```python
from build123d import *

# Parameters (mm, degrees)
SKETCH1_W           = 80
SKETCH1_H           = 40
BOSS_EXTRUDE1_DEPTH = 1.5
SKETCH3_W           = 6.333333333
SKETCH3_H           = 3
SKETCH3_W_2         = 12.666666667
CUT_EXTRUDE1_DEPTH  = 3
CUT_EXTRUDE3_DEPTH  = 3
SKETCH5_W           = 3
SKETCH5_H           = 8
CUT_EXTRUDE4_DEPTH  = 3
CUT_EXTRUDE6_DEPTH  = 3
FILLET1_R           = 3
BOSS_EXTRUDE2_START = -3
BOSS_EXTRUDE2_DEPTH = 3
FILLET2_R           = 6
BOSS_EXTRUDE3_START = -3
BOSS_EXTRUDE3_DEPTH = 3
FILLET3_R           = 1.5


with BuildPart() as part:
    # Sketch1 → Boss-Extrude1 (new body, symmetric)
    with BuildSketch(Plane.XY):
        with Locations((0, 5.625841184)):
            Rectangle(SKETCH1_W, SKETCH1_H)
    extrude(amount=BOSS_EXTRUDE1_DEPTH, both=True)

    # Sketch3 → Cut-Extrude1 (cut)
    with BuildSketch(Plane(origin=(0, 0, -1.5), x_dir=(-1, 0, 0), z_dir=(0, 0, -1))):
        with Locations((-36.833333334, 24.125841184)):
            Rectangle(SKETCH3_W, SKETCH3_H)
        with Locations((-13.333333334, 24.125841184)):
            Rectangle(SKETCH3_W_2, SKETCH3_H)
        with Locations((13.333333334, 24.125841184)):
            Rectangle(SKETCH3_W_2, SKETCH3_H)
        with Locations((36.833333334, 24.125841184)):
            Rectangle(SKETCH3_W, SKETCH3_H)
        with Locations((-36.833333334, -12.874158816)):
            Rectangle(SKETCH3_W, SKETCH3_H)
        with Locations((-13.333333334, -12.874158816)):
            Rectangle(SKETCH3_W_2, SKETCH3_H)
        with Locations((36.833333334, -12.874158816)):
            Rectangle(SKETCH3_W, SKETCH3_H)
        with Locations((13.333333334, -12.874158816)):
            Rectangle(SKETCH3_W_2, SKETCH3_H)
    extrude(amount=-CUT_EXTRUDE1_DEPTH, mode=Mode.SUBTRACT)

    # Sketch4 → Cut-Extrude3 (cut)
    with BuildSketch(Plane(origin=(0, 0, -1.5), x_dir=(-1, 0, 0), z_dir=(0, 0, -1))):
        Polygon((10.933333333, 17.875841184), (12.183333333, 17.875841184), (12.183333333, 15.625841184), (14.483333333, 15.625841184), (14.483333333, 17.875841184), (15.733333333, 17.875841184), (15.733333333, 19.625841184), (14.483333333, 19.625841184), (14.483333333, 22.625841184), (12.183333333, 22.625841184), (12.183333333, 19.625841184), (10.933333333, 19.625841184), align=None)
        Polygon((-12.183333333, 22.625841184), (-14.483333333, 22.625841184), (-14.483333333, 19.625841184), (-15.733333333, 19.625841184), (-15.733333333, 17.875841184), (-14.483333333, 17.875841184), (-14.483333333, 15.625841184), (-12.183333333, 15.625841184), (-12.183333333, 17.875841184), (-10.933333333, 17.875841184), (-10.933333333, 19.625841184), (-12.183333333, 19.625841184), align=None)
        Polygon((-10.933333333, -6.624158816), (-12.183333333, -6.624158816), (-12.183333333, -4.374158816), (-14.483333333, -4.374158816), (-14.483333333, -6.624158816), (-15.733333333, -6.624158816), (-15.733333333, -8.374158816), (-14.483333333, -8.374158816), (-14.483333333, -11.374158816), (-12.183333333, -11.374158816), (-12.183333333, -8.374158816), (-10.933333333, -8.374158816), align=None)
        Polygon((12.183333333, -11.374158816), (14.483333333, -11.374158816), (14.483333333, -8.374158816), (15.733333333, -8.374158816), (15.733333333, -6.624158816), (14.483333333, -6.624158816), (14.483333333, -4.374158816), (12.183333333, -4.374158816), (12.183333333, -6.624158816), (10.933333333, -6.624158816), (10.933333333, -8.374158816), (12.183333333, -8.374158816), align=None)
    extrude(amount=-CUT_EXTRUDE3_DEPTH, mode=Mode.SUBTRACT)

    # Sketch5 → Cut-Extrude4 (cut)
    with BuildSketch(Plane(origin=(0, 0, -1.5), x_dir=(-1, 0, 0), z_dir=(0, 0, -1))):
        with Locations((36.5, -4.374158816)):
            Rectangle(SKETCH5_W, SKETCH5_H)
        with Locations((36.5, 15.625841184)):
            Rectangle(SKETCH5_W, SKETCH5_H)
        with Locations((-36.5, 15.625841184)):
            Rectangle(SKETCH5_W, SKETCH5_H)
        with Locations((-36.5, -4.374158816)):
            Rectangle(SKETCH5_W, SKETCH5_H)
    extrude(amount=-CUT_EXTRUDE4_DEPTH, mode=Mode.SUBTRACT)

    # Sketch7 → Cut-Extrude6 (cut)
    with BuildSketch(Plane.XY.offset(1.5)):
        Polygon((-32, 19.625841184), (-32, -8.374158816), (-18.733333333, -8.374158816), (-18.733333333, -1.374158816), (-7.933333333, -1.374158816), (-7.933333333, -8.374158816), (7.933333333, -8.374158816), (7.933333333, -1.374158816), (18.733333333, -1.374158816), (18.733333333, -8.374158816), (32, -8.374158816), (32, 19.625841184), (18.733333333, 19.625841184), (18.733333333, 12.625841184), (7.933333333, 12.625841184), (7.933333333, 19.625841184), (-7.933333333, 19.625841184), (-7.933333333, 12.625841184), (-18.733333333, 12.625841184), (-18.733333333, 19.625841184), align=None)
    extrude(amount=-CUT_EXTRUDE6_DEPTH, mode=Mode.SUBTRACT)

    # Fillet1
    fillet1_edges = [part.edges().sort_by_distance(p)[0] for p in [
        (-32, 19.625841184, 0),
        (-18.733333333, 19.625841184, 0),
        (-7.933333333, 19.625841184, 0),
        (7.933333333, 19.625841184, 0),
        (18.733333333, 19.625841184, 0),
        (32, 19.625841184, 0),
        (32, -8.374158816, 0),
        (18.733333333, -8.374158816, 0),
        (7.933333333, -8.374158816, 0),
        (-7.933333333, -8.374158816, 0),
        (-18.733333333, -8.374158816, 0),
        (-32, -8.374158816, 0),
    ]]
    fillet(fillet1_edges, radius=FILLET1_R)

    # Sketch8 → Boss-Extrude2 (add)
    with BuildSketch(Plane.XY.offset(1.5).offset(BOSS_EXTRUDE2_START)):
        with BuildLine():
            Line((-18.733333333, 12.625841184), (-7.933333333, 12.625841184))
            ThreePointArc((-7.933333333, 12.625841184), (-10.580065112, 5.625841184), (-7.933333333, -1.374158816))
            Line((-7.933333333, -1.374158816), (-18.733333333, -1.374158816))
            ThreePointArc((-18.733333333, -1.374158816), (-16.086601554, 5.625841184), (-18.733333333, 12.625841184))
        make_face()
        with BuildLine():
            Line((7.933333333, 12.625841184), (18.733333333, 12.625841184))
            ThreePointArc((18.733333333, 12.625841184), (16.086601554, 5.625841184), (18.733333333, -1.374158816))
            Line((18.733333333, -1.374158816), (7.933333333, -1.374158816))
            ThreePointArc((7.933333333, -1.374158816), (10.580065112, 5.625841184), (7.933333333, 12.625841184))
        make_face()
    extrude(amount=BOSS_EXTRUDE2_DEPTH)

    # Fillet2
    fillet2_edges = [part.edges().sort_by_distance(p)[0] for p in [
        (-18.733333333, 12.625841184, 0),
        (-7.933333333, 12.625841184, 0),
        (7.933333333, 12.625841184, 0),
        (18.733333333, 12.625841184, 0),
        (18.733333333, -1.374158816, 0),
        (7.933333333, -1.374158816, 0),
        (-7.933333333, -1.374158816, 0),
        (-18.733333333, -1.374158816, 0),
    ]]
    fillet(fillet2_edges, radius=FILLET2_R)

    # Sketch9 → Boss-Extrude3 (add)
    with BuildSketch(Plane.XY.offset(1.5).offset(BOSS_EXTRUDE3_START)):
        with BuildLine():
            Line((-32, 7.125841184), (-16.193473372, 7.125841184))
            ThreePointArc((-16.193473372, 7.125841184), (-16.086601554, 5.625841184), (-16.193473372, 4.125841184))
            Line((-16.193473372, 4.125841184), (-32, 4.125841184))
            Line((-32, 4.125841184), (-32, 7.125841184))
        make_face()
        with BuildLine():
            Line((-10.473193294, 7.125841184), (10.473193294, 7.125841184))
            ThreePointArc((10.473193294, 7.125841184), (10.580065112, 5.625841184), (10.473193294, 4.125841184))
            Line((10.473193294, 4.125841184), (-10.473193294, 4.125841184))
            ThreePointArc((-10.473193294, 4.125841184), (-10.580065112, 5.625841184), (-10.473193294, 7.125841184))
        make_face()
        with BuildLine():
            Line((16.193473372, 7.125841184), (32, 7.125841184))
            Line((32, 7.125841184), (32, 4.125841184))
            Line((32, 4.125841184), (16.193473372, 4.125841184))
            ThreePointArc((16.193473372, 4.125841184), (16.086601554, 5.625841184), (16.193473372, 7.125841184))
        make_face()
    extrude(amount=BOSS_EXTRUDE3_DEPTH)

    # Fillet3
    fillet3_edges = [part.edges().sort_by_distance(p)[0] for p in [
        (-32, 4.125841184, 0),
        (-32, 7.125841184, 0),
        (-16.193473372, 7.125841184, 0),
        (-16.193473372, 4.125841184, 0),
        (-10.473193294, 4.125841184, 0),
        (-10.473193294, 7.125841184, 0),
        (10.473193294, 7.125841184, 0),
        (10.473193294, 4.125841184, 0),
        (16.193473372, 4.125841184, 0),
        (16.193473372, 7.125841184, 0),
        (32, 7.125841184, 0),
        (32, 4.125841184, 0),
    ]]
    fillet(fillet3_edges, radius=FILLET3_R)


solid = part.part
```
CAD build for the part. Positions are in the model's coordinates, mm. A direction names the side the tool comes from. Round coordinates to 2 decimals unless told otherwise and drop trailing zeros. Write each loop counter-clockwise with the first axis right and the second up, starting at its lowest first coordinate (ties: lowest second). Pieces come first, ordered by that corner, then holes. Notation, with made-up numbers: (-23.75, 24) -> (-2.75, 24) arc R32 cw to (-2.75, 53) -> close; hole circle Ø4 at (75.25, 41.25). An arc over 180 degrees is marked (long way). Answer in a Markdown table with one row per item. Add a question column.
Item 1: Saw through at B-B, the plane z = 0.75. Count the separate pieces of the cut face and the enclosed holes in it, then the cut area to 3 significant figures.
Item 2: Saw through at C-C, the plane x = -13.5. Write the cut outline in (y, z), then the cut area to 3 significant figures.
Item 3: Drop flat-ended pins along their axis: pin 1 Ø0.9 at (x, z) = (-35.5, 0.5) entering from +Y; pin 2 Ø0.9 at (x, z) = (17.5, 0.5) entering from -Y. Give the stop position or say it passes through.
Item 4: Which spindle directions (+Z, -Z, +X, -X, +Y, -Y) get a long thin tool onto all of the face, cutting with end or side? Do faces 1 (the face through (-7, 24, 0)), 2 (the face through (-27, -14.374, 0)), 3 (the face through (7.933, 16, 0)). Say none if no direction does.
Item 5: Mould opens along X. For faces 4 (the face through (37, -11.374, 0)), 5 (the face through (-33.667, 24, 0)), 6 (the face through (-10.933, 19, 0)) say: pulls with the +X half, pulls with the -X half, needs draft (parallel to the pull), parting line crosses it, or undercut.
Item 6: Drill centre lines: line 1 (Y direction, x = 0, z = 0.05); line 2 (X direction, y = -12, z = -1.2); line 3 (Y direction, x = -12, z = -1.3). Where is each one in solid material? Low to high. Write a range as from..to.
Item 7: Saw through at A-A, the plane x = -24.5. Write the cut outline in (y, z).
Findings below:
| question | item | result |
|---|---|---|
| 1 | separate pieces | 1 |
| 1 | enclosed holes | 10 |
| 1 | area | 1,690 mm^2 |
| 2 | outline | (-4.37, -1.5) -> (15.63, -1.5) -> (15.63, 1.5) -> (-4.37, 1.5) -> close |
| 2 | area | 60.0 mm^2 |
| 3 | pin 1 | stops at y = 22.63 |
| 3 | pin 2 | stops at y = -11.37 |
| 4 | face 1 | +Z, -Z, +Y |
| 4 | face 2 | +Z, -Z, +X, -X, -Y |
| 4 | face 3 | +Z, -Z |
| 5 | face 4 | needs draft |
| 5 | face 5 | pulls with the -X half |
| 5 | face 6 | undercut |
| 6 | line 1 | y = -14.37..-8.37, 4.13..7.13, 19.63..25.63 |
| 6 | line 2 | x = -33.67..-19.67, -7..7, 19.67..33.67 |
| 6 | line 3 | y = -11.37..-8.37, -6.62..17.88, 19.63..22.63 |
| 7 | outline | (-14.37, -1.5) -> (-8.37, -1.5) -> (-8.37, 1.5) -> (-14.37, 1.5) -> close; (4.13, -1.5) -> (7.13, -1.5) -> (7.13, 1.5) -> (4.13, 1.5) -> close; (19.63, -1.5) -> (25.63, -1.5) -> (25.63, 1.5) -> (19.63, 1.5) -> close |
